```python
from build123d import *

# Parameters (mm, degrees)
EXTRUDE_1_DEPTH   = 2
HOLE_WIZARD_M61_D = 6.6
CHAMFER_1_SIZE    = 2


with BuildPart() as part:
    # Эскиз1 → Бобышка-Вытянуть1 (new body)
    with BuildSketch(Plane(origin=(0, 0, 0), x_dir=(1, 0, 0), z_dir=(0, 0, -1))):
        Polygon((0, 0), (0, 90), (60, 90), (60, 60), (30, 60), (30, 0), align=None)
    extrude(amount=EXTRUDE_1_DEPTH)

    # Отверстие с зазором M61 (through all)
    with Locations(Plane(origin=(0, 0, -2), x_dir=(1, 0, 0), z_dir=(0, 0, -1))):
        with Locations((45, 75), (15, 75), (15, 45), (15, 15)):
            Hole(HOLE_WIZARD_M61_D / 2)

    # Фаска1
    chamfer_1_edges = [part.edges().sort_by_distance(p)[0] for p in [
        (0, 0, -1),
        (0, -90, -1),
        (60, -90, -1),
        (60, -60, -1),
        (30, 0, -1),
    ]]
    chamfer(chamfer_1_edges, length=CHAMFER_1_SIZE)


solid = part.part
```
CAD build for the part. Positions are in the model's coordinates, mm. A direction names the side the tool comes from. Round coordinates to 2 decimals unless told otherwise and drop trailing zeros. Order: outer loops, then holes, each group sorted by start corner. A loop starts at its lowest first (then second) coordinate and runs counter-clockwise, first axis right, second up. Notation, with made-up numbers: (-0.5, 7.25) - (51.5, 7.25) arc R15 cw to (51.5, 22.25) - close; hole circle Ø8 at (7.25, 84.5). An arc over 180 degrees is marked (long way). Answer in a Markdown table with one row per item. Add a question column.
(1) Mould opens along Y. For faces 3 (the face through (1, -89, -1)), 4 (the face through (15.43, -48.27, -0.99)), 5 (the face through (0, -44, -1)) say: +Y half, -Y half, draft (parallel to the pull), parting line (faces both ways), or undercut.
(2) 3-axis set-ups, long thin cutter, end or side, ignore diameter. For faces 1 (the face through (44, -60, -1)), 2 (the face through (18.3, -15.1, -1)): which of +Z, -Z, +X, -X, +Y, -Y reach the whole face in a straight line?
(3) Band-saw the part on D-D on z = -0.55. List the corners of the cut face in (x, y), and give its area (3 significant figures).
(4) Probe L1, parallel to Y at x = 15, z = -1.45; L2, parallel to X at y = -75, z = -0.8; L3, parallel to X at y = -15, z = -1.5. List the from-to ranges inside material, lowest first. Write a range as [from, to].
(5) Band-saw the part on B-B on y = -45. List the corners of the cut face in (x, z).
(6) Band-saw the part on C-C on x = 45. List the corners of the cut face in (y, z), and give its area (3 significant figures).
(7) Drop a flat-ended pin along its axis: pin 1 Ø4 at (x, y) = (15, -15) entering from +Z. Give the stop position or say it passes through.
(8) Band-saw the part on A-A on y = -75. List the corners of the cut face in (x, z), and give its area (3 significant figures).
Data:
| question | item | result |
|---|---|---|
| 1 | face 3 | -Y half |
| 1 | face 4 | undercut |
| 1 | face 5 | draft |
| 2 | face 1 | +Z, -Z, +X, +Y |
| 2 | face 2 | +Z, -Z |
| 3 | outline | (0, -88) - (2, -90) - (58, -90) - (60, -88) - (60, -62) - (58, -60) - (30, -60) - (30, -2) - (28, 0) - (2, 0) - (0, -2) - close; hole circle Ø6.6 at (15, -75); hole circle Ø6.6 at (15, -45); hole circle Ø6.6 at (15, -15); hole circle Ø6.6 at (45, -75) |
| 3 | area | 3,450 mm^2 |
| 4 | L1 | y = [-90, -78.3], [-71.7, -48.3], [-41.7, -18.3], [-11.7, 0] |
| 4 | L2 | x = [0, 11.7], [18.3, 41.7], [48.3, 60] |
| 4 | L3 | x = [0, 11.7], [18.3, 30] |
| 5 | outline | (0, -2) - (11.7, -2) - (11.7, 0) - (0, 0) - close; (18.3, -2) - (30, -2) - (30, 0) - (18.3, 0) - close |
| 6 | outline | (-90, -2) - (-78.3, -2) - (-78.3, 0) - (-90, 0) - close; (-71.7, -2) - (-60, -2) - (-60, 0) - (-71.7, 0) - close |
| 6 | area | 46.8 mm^2 |
| 7 | pin 1 | passes through |
| 8 | outline | (0, -2) - (11.7, -2) - (11.7, 0) - (0, 0) - close; (18.3, -2) - (41.7, -2) - (41.7, 0) - (18.3, 0) - close; (48.3, -2) - (60, -2) - (60, 0) - (48.3, 0) - close |
| 8 | area | 93.6 mm^2 |
